```python
from build123d import *

# Parameters (mm, degrees)
SKETCH004_W     = 114
SKETCH004_H     = 5
PAD001_DEPTH    = 10
SKETCH005_R     = 1.43
POCKET003_DEPTH = 10
CHAMFER_SIZE    = 0.8
SKETCH009_R     = 2.75
SKETCH009_R_2   = 1.43
POCKET006_DEPTH = 5


with BuildPart() as part:
    # Sketch004 → Pad001 (new body)
    with BuildSketch(Plane.XY):
        with Locations((60, 45)):
            Rectangle(SKETCH004_W, SKETCH004_H)
    extrude(amount=PAD001_DEPTH)

    # Sketch005 (on Face6 of Pad001) → Pocket003 (cut)
    with BuildSketch(Plane.XY.offset(10)):
        with Locations((8, 45)):
            Circle(SKETCH005_R)
        with Locations((112, 45)):
            Circle(SKETCH005_R)
    extrude(amount=-POCKET003_DEPTH, mode=Mode.SUBTRACT)

    # Chamfer
    chamfer_edges = [part.edges().sort_by_distance(p)[0] for p in [
        (110.57, 45, 10),
        (6.57, 45, 10),
    ]]
    chamfer(chamfer_edges, length=CHAMFER_SIZE)

    # Sketch009 (on Face6 of Chamfer) → Pocket006 (cut)
    with BuildSketch(Plane.XZ.offset(-42.5)):
        with Locations((45, 5)):
            Circle(SKETCH009_R)
        with Locations((75, 5)):
            Circle(SKETCH009_R_2)
    extrude(amount=-POCKET006_DEPTH, mode=Mode.SUBTRACT)


with BuildPart() as part_1:
    # Body001 placement: moved
    add(part.part.moved(Location((0, 0, 8))))


solid = part_1.part
```
Geometry check sheet. Reference: the model listing, model coordinates, mm. Give positions to 0.01 mm unless a question says otherwise; leave off trailing zeros. Order: outer loops, then holes, each group sorted by start corner. A loop starts at its lowest first (then second) coordinate and runs counter-clockwise, first axis right, second up.
1. Section check A-A, the plane z = 13. Enter the section's corners in (x, y).
2. Thickness scan on L1, parallel to Z at x = 75, y = 45.15; L2, parallel to Y at x = 112, z = 14.5; L3, parallel to Z at x = 45, y = 43.7. Record the ranges inside material, lowest first.
3. Release check for a two-part mould opening along Y. For faces 1 (the face through (59, 47.5, 13)), 2 (the face through (113.364, 45.43, 12.664)), 3 (the face through (59, 42.5, 13)) record: pulls with the +Y half, pulls with the -Y half, needs draft (parallel to the pull), parting line crosses it, or undercut.
4. Section check C-C, the plane x = 45. Enter the section's corners in (y, z).
5. Section check B-B, the plane y = 45. Enter the section's corners in (x, z), and give its area (3 significant figures).
6. Section check D-D, the plane x = 112. Enter the section's corners in (y, z).
Values follow:
1. outline: (3, 42.5) - (42.25, 42.5) - (42.25, 47.5) - (3, 47.5) - close; (47.75, 42.5) - (73.57, 42.5) - (73.57, 47.5) - (47.75, 47.5) - close; (76.43, 42.5) - (117, 42.5) - (117, 47.5) - (76.43, 47.5) - close; hole circle Ø2.86 at (8, 45); hole circle Ø2.86 at (112, 45)
2. L1: z = 8 to 11.57, 14.43 to 18
2. L2: y = 42.5 to 43.57, 46.43 to 47.5
2. L3: z = 8 to 10.25, 15.75 to 18
3. face 1: pulls with the +Y half
3. face 2: undercut
3. face 3: pulls with the -Y half
4. outline: (42.5, 8) - (47.5, 8) - (47.5, 10.25) - (42.5, 10.25) - close; (42.5, 15.75) - (47.5, 15.75) - (47.5, 18) - (42.5, 18) - close
5. outline: (3, 8) - (6.57, 8) - (6.57, 17.2) - (5.77, 18) - (3, 18) - close; (9.43, 8) - (110.57, 8) - (110.57, 17.2) - (109.77, 18) - (10.23, 18) - (9.43, 17.2) - close; (113.43, 8) - (117, 8) - (117, 18) - (114.23, 18) - (113.43, 17.2) - close; hole circle Ø5.5 at (45, 13); hole circle Ø2.86 at (75, 13)
5. area: 1,050 mm2
6. outline: (42.5, 8) - (43.57, 8) - (43.57, 17.2) - (42.77, 18) - (42.5, 18) - close; (46.43, 8) - (47.5, 8) - (47.5, 18) - (47.23, 18) - (46.43, 17.2) - close
